Check sheet for the modelled part. Datum: model origin and axes. Units: mm. A direction names the side the tool comes from. Give positions to 0.01 mm unless a question says otherwise; leave off trailing zeros. Write each loop counter-clockwise with the first axis right and the second up, starting at its lowest first coordinate (ties: lowest second). Pieces come first, ordered by that corner, then holes. Notation, with made-up numbers: (6, -29.75) -> (22, -29.75) arc R20 ccw to (22, -19.75) -> close; hole circle Ø10 at (86.5, 39.5). An arc over 180 degrees is marked (long way). Answer as a JSON object with one key per item and string values.
from build123d import *

# Parameters (mm, degrees)
F0_W     = 25.4
F0_H     = 25.4
F1_DEPTH = 25.4
F5_DEPTH = 2.54
F6_DEPTH = 2.54
F7_DEPTH = 2.54


with BuildPart() as f1:
    # F0 (on Top) → F1 (new body)
    with BuildSketch(Plane.XY):
        Rectangle(F0_W, F0_H)
    extrude(amount=F1_DEPTH)

    # F2 (on face) → F5 (join)
    with BuildSketch(Plane.XY.offset(25.4)):
        with BuildLine():
            ThreePointArc((12.7, 0), (8.980256, 8.980256), (0, 12.7))
            Line((0, 12.7), (-12.7, 12.7))
            Line((-12.7, 12.7), (-12.7, -12.7))
            Line((-12.7, -12.7), (0, -12.7))
            ThreePointArc((0, -12.7), (8.980256, -8.980256), (12.7, 0))
        make_face()
        with BuildLine():
            Line((-6.35, -6.35), (-6.35, 6.35))
            Line((-6.35, 6.35), (0, 6.35))
            ThreePointArc((0, 6.35), (4.490128, 4.490128), (6.35, 0))
            ThreePointArc((6.35, 0), (4.490128, -4.490128), (0, -6.35))
            Line((0, -6.35), (-6.35, -6.35))
        make_face(mode=Mode.SUBTRACT)
    extrude(amount=F5_DEPTH)

    # F3 (on face) → F6 (join)
    with BuildSketch(Plane.XZ.offset(12.7)):
        with BuildLine():
            Line((-12.7, 25.4), (-12.7, 0))
            Line((-12.7, 0), (0, 0))
            ThreePointArc((0, 0), (8.980256, 3.719744), (12.7, 12.7))
            ThreePointArc((12.7, 12.7), (8.980256, 21.680256), (0, 25.4))
            Line((0, 25.4), (-12.7, 25.4))
        make_face()
        with BuildLine():
            Line((-6.35, 19.05), (0, 19.05))
            ThreePointArc((0, 19.05), (4.490128, 17.190128), (6.35, 12.7))
            ThreePointArc((6.35, 12.7), (4.490128, 8.209872), (0, 6.35))
            Line((0, 6.35), (-6.35, 6.35))
            Line((-6.35, 6.35), (-6.35, 19.05))
        make_face(mode=Mode.SUBTRACT)
    extrude(amount=F6_DEPTH)

    # F4 (on face) → F7 (cut)
    with BuildSketch(Plane.YZ.offset(12.7)):
        with BuildLine():
            Line((0, 19.05), (-6.35, 19.05))
            Line((-6.35, 19.05), (-6.35, 6.35))
            Line((-6.35, 6.35), (0, 6.35))
            ThreePointArc((0, 6.35), (4.490128, 8.209872), (6.35, 12.7))
            ThreePointArc((6.35, 12.7), (4.490128, 17.190128), (0, 19.05))
        make_face()
        with BuildLine():
            Line((12.7, 25.4), (0, 25.4))
            ThreePointArc((0, 25.4), (8.980256, 21.680256), (12.7, 12.7))
            Line((12.7, 12.7), (12.7, 25.4))
        make_face()
        with BuildLine():
            Line((12.7, 0), (12.7, 12.7))
            ThreePointArc((12.7, 12.7), (8.980256, 3.719744), (0, 0))
            Line((0, 0), (12.7, 0))
        make_face()
    extrude(amount=-F7_DEPTH, mode=Mode.SUBTRACT)


solid = f1.part
1. Go/stop test with flat-tipped pins: P1, Ø3, axis at x = -9, y = -13.5, coming from the +Z side; P2, Ø1.3, axis at x = 12, y = 3.5, coming from the -Z side; P3, Ø4, axis at x = -0.5, z = 11.5, coming from the -Y side. Record where each tip stops, or that it passes through.
Determined:
{"P1": "z = 27.94", "P2": "z = 0.32", "P3": "y = -12.7"}
2. Access from +Z, -Z, +X, -X, +Y, -Y to the whole of each face (thin tool, end or side, straight path). Record for faces 5 (the face through (10, -12.7, 23)), 6 (the face through (10.16, 10, 23)), 7 (the face through (0, 0, 25.4)).
Determined:
{"face 5": "+Z, +X, -Y", "face 6": "+X, +Y", "face 7": "+Z"}
3. Mould release check, pull along X, two halves, no side actions. Record for faces 1 (the face through (-3, -6.35, 27)), 2 (the face through (-3, -14, 19.05)), 3 (the face through (-1, 12.7, 14)), 4 (the face through (-12.7, -1, 14)): released by +X, released by -X, zero draft, split by the parting line, or undercut.
Determined:
{"face 1": "undercut", "face 2": "undercut", "face 3": "zero draft", "face 4": "released by -X"}
4. Sectioned sample at D-D, the plane x = 10.75. Enter the section's corners in (y, z), plus the area to 3 significant figures.
Determined:
{"outline": "(-15.24, 5.94) -> (-12.7, 5.94) -> (-12.7, 0) -> (0, 0) arc R12.7 ccw to (0, 25.4) -> (6.76, 25.4) -> (6.76, 27.94) -> (-6.76, 27.94) -> (-6.76, 25.4) -> (-12.7, 25.4) -> (-12.7, 19.46) -> (-15.24, 19.46) -> close; hole (-6.35, 6.35) -> (0, 6.35) arc R6.35 ccw to (0, 19.05) -> (-6.35, 19.05) -> close", "area": "501 mm^2"}
5. Sectioned sample at B-B, the plane z = 11.5. Enter the section's corners in (x, y), plus the area to 3 significant figures.
Determined:
{"outline": "(-12.7, -15.24) -> (-6.35, -15.24) -> (-6.35, -12.7) -> (6.24, -12.7) -> (6.24, -15.24) -> (12.64, -15.24) -> (12.64, -12.7) -> (12.7, -12.7) -> (12.7, -6.35) -> (10.16, -6.35) -> (10.16, 6.24) -> (12.7, 6.24) -> (12.7, 12.64) -> (10.16, 12.64) -> (10.16, 12.7) -> (-12.7, 12.7) -> close", "area": "645 mm^2"}
6. Scan lines: L1, parallel to Y at x = -1, z = 26.5; L2, parallel to Y at x = 1.75, z = 15.5; L3, parallel to Z at x = 11.25, y = 4.5. Record each from-to range of solid material in increasing order. Write a range as [from, to].
Determined:
{"L1": "[-12.7, -6.35], [6.35, 12.7]", "L2": "[-12.7, 12.7]", "L3": "[0.82, 8.22], [17.18, 24.58], [25.4, 27.94]"}
7. Sectioned sample at C-C, the plane y = -2.75. Enter the section's corners in (x, z), plus the area to 3 significant figures.
Determined:
{"outline": "(-12.7, 0) -> (12.7, 0) -> (12.7, 6.35) -> (10.16, 6.35) -> (10.16, 19.05) -> (12.7, 19.05) -> (12.7, 25.4) -> (12.4, 25.4) -> (12.4, 27.94) -> (5.72, 27.94) -> (5.72, 25.4) -> (-6.35, 25.4) -> (-6.35, 27.94) -> (-12.7, 27.94) -> close", "area": "646 mm^2"}
8. Sectioned sample at A-A, the plane x = -1.5. Enter the section's corners in (y, z), plus the area to 3 significant figures.
Determined:
{"outline": "(-15.24, 0) -> (12.7, 0) -> (12.7, 27.94) -> (6.35, 27.94) -> (6.35, 25.4) -> (-6.35, 25.4) -> (-6.35, 27.94) -> (-12.7, 27.94) -> (-12.7, 25.4) -> (-15.24, 25.4) -> (-15.24, 19.05) -> (-12.7, 19.05) -> (-12.7, 6.35) -> (-15.24, 6.35) -> close", "area": "710 mm^2"}
